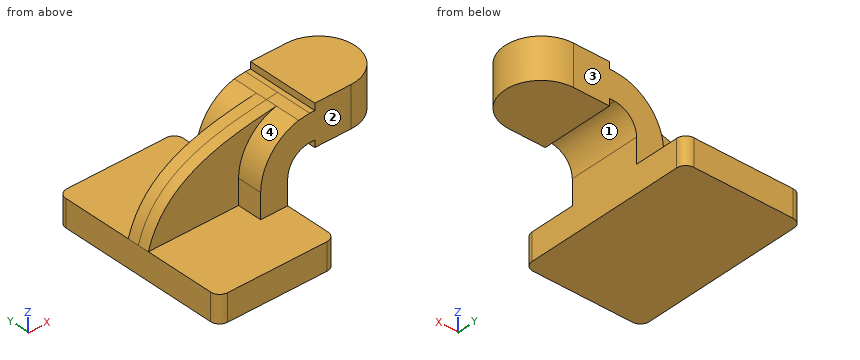
```python
from build123d import *

# Parameters (mm, degrees)
F1_DEPTH = 63.5
F2_DEPTH = 25.4
F3_DEPTH = 7.9375
F0_W     = 25.4
F0_H     = 28.575
F5_R     = 6.35


with BuildPart() as f1:
    # F0 (on Front) → F1 (new body, symmetric)
    with BuildSketch(Plane.XZ):
        Polygon((41.275, -9.525), (41.275, 9.525), (22.225, 9.525), (-41.275, 9.525), (-41.275, -9.525), align=None)
    extrude(amount=F1_DEPTH, both=True)

    # F0 (on Front) → F2 (join, symmetric)
    with BuildSketch(Plane.XZ):
        with BuildLine():
            Line((22.225, 9.525), (41.275, 9.525))
            Line((41.275, 9.525), (41.275, 27.00272))
            ThreePointArc((41.275, 27.00272), (45.825119, 38.127588), (56.867151, 42.8752))
            Line((56.867151, 42.8752), (60.325, 42.8752))
            Line((60.325, 42.8752), (60.325, 61.9252))
            Line((60.325, 61.9252), (56.730458, 61.9252))
            add(Edge.make_bspline(
                [(48.933699, 60.947499), (51.581091, 61.280162), (54.185468, 61.601631), (56.730458, 61.9252)],
                knots=[103.418833, 103.418833, 103.418833, 103.418833, 111.134381, 111.134381, 111.134381, 111.134381], degree=3))
            ThreePointArc((48.933699, 60.947499), (29.702687, 48.599031), (22.225, 27.00272))
            Line((22.225, 27.00272), (22.225, 9.525))
        make_face()
        Polygon((60.325, 61.9252), (60.325, 42.8752), (60.325, 38.1), (85.725, 38.1), (85.725, 66.675), (60.325, 66.675), align=None)
    extrude(amount=F2_DEPTH, both=True)

    # F0 (on Front) → F3 (join, symmetric)
    with BuildSketch(Plane.XZ):
        with BuildLine():
            Line((-41.275, 9.525), (22.225, 9.525))
            Line((22.225, 9.525), (22.225, 27.00272))
            ThreePointArc((22.225, 27.00272), (29.702687, 48.599031), (48.933699, 60.947499))
            add(Edge.make_bspline(
                [(-41.275, 9.525), (-29.76549, 50.018415), (13.44819, 56.488502), (48.933699, 60.947499)],
                knots=[0, 0, 0, 0, 103.418833, 103.418833, 103.418833, 103.418833], degree=3))
        make_face()
    extrude(amount=F3_DEPTH, both=True)

    # F0 (on Front) → F4 (revolve)
    with BuildSketch(Plane.XZ):
        with Locations((98.425, 52.3875)):
            Rectangle(F0_W, F0_H)
    revolve(axis=Axis((85.725, 0, 52.3875), (0, 0, -1)))

    # F5
    f5_edges = [f1.edges().sort_by_distance(p)[0] for p in [
        (-41.275, -63.5, 0),
        (41.275, -63.5, 0),
        (41.275, 63.5, 0),
        (-41.275, 63.5, 0),
    ]]
    fillet(f5_edges, radius=F5_R)


solid = f1.part
```
Build history of the part. All positions in model axes, mm. Face numbers are marked on the shaded views. A direction names the side the tool comes from. Round coordinates to 2 decimals unless told otherwise and drop trailing zeros. Write each loop counter-clockwise with the first axis right and the second up, starting at its lowest first coordinate (ties: lowest second). Pieces come first, ordered by that corner, then holes.
1) 3-axis set-ups, long thin cutter, end or side, ignore diameter. For the marked faces 1, 2, 3 and 4: which of +Z, -Z, +X, -X, +Y, -Y reach the whole face in a straight line?
2) Band-saw the part on C-C, the plane y = 42.5. List the corners of the cut face in (x, z) (3 decimals), and give its area (3 significant figures).
3) Drill centre lines: probe 1 along Y at (x, z) = (17.5, 31.5); probe 2 along X at (y, z) = (-15, 14.5) (3 decimals); probe 3 along Z at (x, y) = (14, -57.5) (3 decimals). Where is each one in solid material? Low to high.
4) Band-saw the part on A-A, the plane z = 4.5. List the corners of the cut face in (x, y) (3 decimals), and give its area (3 significant figures).
5) Pin check, flat tips, straight feed: pin 1 (15.5 mm diameter, centred on x = 9.5, z = 24, fed in from -Y); pin 2 (1.1 mm diameter, centred on x = 58, y = -9, fed in from +Z); pin 3 (1.5 mm diameter, centred on x = -7.5, z = 15, fed in from +Y). Stop position of each tip, or through.
6) Band-saw the part on B-B, the plane x = 79. List the corners of the cut face in (y, z) (3 decimals), and give its area (3 significant figures).
Ans:
1. face 1: -Z, +Y, -Y
1. face 2: +Z, +X, -X, -Y
1. face 3: +Z, +X, -X, +Y
1. face 4: +Z, -X, -Y
2. outline: (-41.275, -9.525) - (41.275, -9.525) - (41.275, 9.525) - (-41.275, 9.525) - close
2. area: 1,570 mm2
3. probe 1: y = -7.94 to 7.94
3. probe 2: x = 22.225 to 41.275
3. probe 3: z = -9.525 to 9.525
4. outline: (-41.275, -57.15) arc R6.35 ccw to (-34.925, -63.5) - (34.925, -63.5) arc R6.35 ccw to (41.275, -57.15) - (41.275, 57.15) arc R6.35 ccw to (34.925, 63.5) - (-34.925, 63.5) arc R6.35 ccw to (-41.275, 57.15) - close
4. area: 10,400 mm2
5. pin 1: stops at y = -7.94
5. pin 2: stops at z = 61.93
5. pin 3: stops at y = 7.94
6. outline: (-25.4, 38.1) - (25.4, 38.1) - (25.4, 66.675) - (-25.4, 66.675) - close
6. area: 1,450 mm2
